Source: CAD feature listing. Evaluate the final solid. Frame: model axes, mm. Face numbers are marked on the shaded views. Give positions to 0.01 mm unless a question says otherwise; leave off trailing zeros. Write each loop counter-clockwise with the first axis right and the second up, starting at its lowest first coordinate (ties: lowest second). Pieces come first, ordered by that corner, then holes. Notation, with made-up numbers: M -33.75,83 L 3.25,83 A17 cw 3.25,99 Z; hole C 27.25,60 d11. An arc over 180 degrees is marked long. Return JSON: item names as keys, results as strings.
```python
from build123d import *

# Parameters (mm, degrees)
SKETCH1_R                     = 15
BOSS_EXTRUDE1_DEPTH           = 65
FILLET1_R                     = 2
FILLET2_R                     = 1
SKETCH2_R                     = 2
BOSS_EXTRUDE2_DEPTH           = 5
BOSS_EXTRUDE2_DRAFT           = 16
BOSS_EXTRUDE2_PROFILE_2_DEPTH = 5
BOSS_EXTRUDE2_PROFILE_2_DRAFT = 16


with BuildPart() as part:
    # Sketch1 → Boss-Extrude1 (new body)
    with BuildSketch(Plane(origin=(0, 0, 0), x_dir=(1, 0, 0), z_dir=(0, 1, 0))):
        with Locations(Location((0, 0, 0), (0, 0, 270))):
            Circle(SKETCH1_R)
    extrude(amount=BOSS_EXTRUDE1_DEPTH)

    # Fillet1
    fillet1_edges = [part.edges().sort_by_distance(p)[0] for p in [
        (0, 65, -15),
    ]]
    fillet(fillet1_edges, radius=FILLET1_R)

    # Fillet2
    fillet2_edges = [part.edges().sort_by_distance(p)[0] for p in [
        (0, 0, -15),
    ]]
    fillet(fillet2_edges, radius=FILLET2_R)


with BuildPart() as boss_extrude2_tool:
    # Sketch2 → Boss-Extrude2 (with draft: the straight prism first)
    with BuildSketch(Plane(origin=(0, 0, 0), x_dir=(-1, 0, 0), z_dir=(0, -1, 0))):
        with Locations((6, 0)):
            Circle(SKETCH2_R)
    extrude(amount=BOSS_EXTRUDE2_DEPTH)
    # Boss-Extrude2: the draft: its side faces are tilted about the plane it starts from
    boss_extrude2_sides = [boss_extrude2_tool.faces().sort_by_distance(p)[0] for p in [
        (-4, -2.5, 0),
    ]]
    draft(boss_extrude2_sides, Plane(origin=(0, 0, 0), x_dir=(-1, 0, 0), z_dir=(0, -1, 0)), BOSS_EXTRUDE2_DRAFT)


with BuildPart() as part_1:
    add(part.part)

    # Boss-Extrude2: add boss_extrude2_tool
    add(boss_extrude2_tool.part)


with BuildPart() as boss_extrude2_profile_2_tool:
    # Sketch2 → Boss-Extrude2 profile 2 (with draft: the straight prism first)
    with BuildSketch(Plane(origin=(0, 0, 0), x_dir=(-1, 0, 0), z_dir=(0, -1, 0))):
        with Locations((-6, 0)):
            Circle(SKETCH2_R)
    extrude(amount=BOSS_EXTRUDE2_PROFILE_2_DEPTH)
    # Boss-Extrude2 profile 2: the draft: its side faces are tilted about the plane it starts from
    boss_extrude2_profile_2_sides = [boss_extrude2_profile_2_tool.faces().sort_by_distance(p)[0] for p in [
        (8, -2.5, 0),
    ]]
    draft(boss_extrude2_profile_2_sides, Plane(origin=(0, 0, 0), x_dir=(-1, 0, 0), z_dir=(0, -1, 0)), BOSS_EXTRUDE2_PROFILE_2_DRAFT)


with BuildPart() as part_2:
    add(part_1.part)

    # Boss-Extrude2 profile 2: add boss_extrude2_profile_2_tool
    add(boss_extrude2_profile_2_tool.part)


solid = part_2.part
```
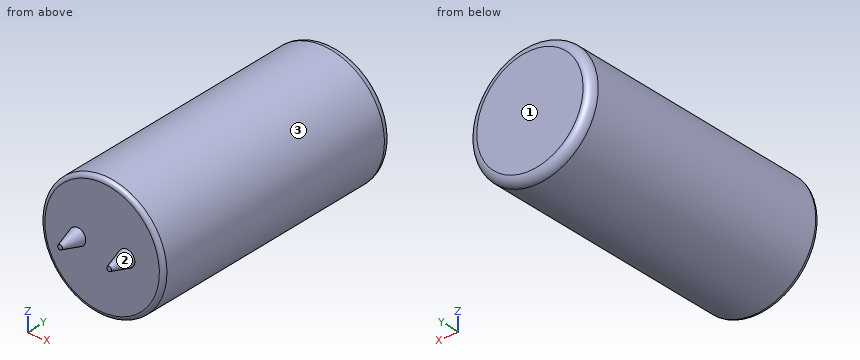
1) Cut plane B-B, the plane y = 6.5. Return the cut outline in (x, z), then the cut area to 3 significant figures.
Numbers:
{"outline": "C 0,0 d30", "area": "707 mm²"}
2) Cut plane A-A, the plane x = 0. Return the cut outline in (y, z), then the cut area to 3 significant figures.
Numbers:
{"outline": "M 0,-14 A1 ccw 1,-15 L 63,-15 A2 ccw 65,-13 L 65,13 A2 ccw 63,15 L 1,15 A1 ccw 0,14 Z", "area": "1,950 mm²"}
3) Line query: line 1 (Y direction, x = -0.75, z = -8); line 2 (Z direction, x = -9.5, y = 44); line 3 (X direction, y = 11, z = -13.25). Output: solid intervals per line, ascending. Write a range as [from, to].
Numbers:
{"line 1": "y = [0, 65]", "line 2": "z = [-11.61, 11.61]", "line 3": "x = [-7.03, 7.03]"}
4) Draft query along X for the marked faces 1, 2 and 3. Return one class per face: released by +X, released by -X, zero draft, split by the parting line, or undercut.
Numbers:
{"face 1": "zero draft", "face 2": "undercut", "face 3": "split by the parting line"}
5) Contact query for flat-ended pins moving along their axis: pin 1 Ø8 at (x, y) = (-11, 48.5) entering from -Z; pin 2 Ø3 at (y, z) = (21.5, 10.5) entering from -X; pin 3 Ø10 at (y, z) = (4, -11) entering from +X; pin 4 Ø12 at (x, y) = (-6, 5.5) entering from -Z. Output: stop coordinate, or through.
Numbers:
{"pin 1": "stops at z = -13.27", "pin 2": "stops at x = -12", "pin 3": "stops at x = 13.75", "pin 4": "stops at z = -15"}
